```python
from build123d import *

# Parameters (mm, degrees)
BOSS_EXTRUDE2_DEPTH  = 18.5
M3_CLEARANCE_HOLE1_D = 3.2
BOSS_EXTRUDE3_REACH  = 43.692
CUT_EXTRUDE1_REACH   = 43.692
FILLET1_R            = 2
FILLET2_R            = 1


# Some blends are built 0.0001 mm under size
with BuildPart() as part:
    # Sketch2 → Boss-Extrude2 (new, symmetric)
    with BuildSketch(Plane.XY):
        with BuildLine():
            Line((-8, 0), (-8, -9))
            Line((-8, -9), (-16, -9))
            Line((-16, -9), (-16, -7))
            Line((-16, -7), (-10, -7))
            Line((-10, -7), (-10, 0))
            ThreePointArc((-10, 0), (0, 10), (10, 0))
            Line((10, 0), (10, -7))
            Line((10, -7), (16, -7))
            Line((16, -7), (16, -9))
            Line((16, -9), (8, -9))
            Line((8, -9), (8, 0))
            ThreePointArc((8, 0), (0, 8), (-8, 0))
        make_face()
    extrude(amount=BOSS_EXTRUDE2_DEPTH, both=True)

    # M3 Clearance Hole1 (through all)
    with Locations(Plane(origin=(0, -7, 0), x_dir=(1, 0, 0), z_dir=(0, 1, 0))):
        with Locations((-13, 14.25), (13, 14.25), (13, -14.25), (-13, -14.25)):
            Hole(M3_CLEARANCE_HOLE1_D / 2)

    # Sketch6 → Boss-Extrude3 (add, up to next)
    with BuildSketch(Plane(origin=(20, 0, 0), x_dir=(0, 0, -1), z_dir=(1, 0, 0)), mode=Mode.PRIVATE) as boss_extrude3_sk1:
        with BuildLine():
            Line((-8, 0), (-8, -9))
            Line((-8, -9), (-10, -9))
            Line((-10, -9), (-10, 0))
            ThreePointArc((-10, 0), (0, 10), (10, 0))
            Line((10, 0), (10, -9))
            Line((10, -9), (8, -9))
            Line((8, -9), (8, 0))
            ThreePointArc((8, 0), (0, 8), (-8, 0))
        make_face()
    boss_extrude3_tool1 = extrude(boss_extrude3_sk1.sketch, amount=-BOSS_EXTRUDE3_REACH, mode=Mode.PRIVATE) - part.part
    add(boss_extrude3_tool1.solids().sort_by_distance((20, -4.5, -9.724138))[0])

    # Sketch7 → Cut-Extrude1 (cut, up to next)
    with BuildSketch(Plane(origin=(20, 0, 0), x_dir=(0, 0, -1), z_dir=(1, 0, 0)), mode=Mode.PRIVATE) as cut_extrude1_sk1:
        with BuildLine():
            Line((8, 0), (8, -7))
            Line((8, -7), (8, -9))
            Line((8, -9), (-8, -9))
            Line((-8, -9), (-8, -7))
            Line((-8, -7), (-8, 0))
            ThreePointArc((-8, 0), (0, 8), (8, 0))
        make_face()
    cut_extrude1_tool1 = extrude(cut_extrude1_sk1.sketch, amount=-CUT_EXTRUDE1_REACH, mode=Mode.PRIVATE) & part.part
    add(cut_extrude1_tool1.solids().sort_by_distance((20, -1.254102, 0))[0], mode=Mode.SUBTRACT)

    # Fillet1
    fillet1_edges = [part.edges().sort_by_distance(p)[0] for p in [
        (16, -8, -10),
        (16, -8, 10),
        (16, -8, 18.5),
        (16, -8, -18.5),
        (-16, -8, 18.5),
        (-16, -8, -18.5),
        (20, -4.5, 10),
        (20, 10, 0),
        (20, -4.5, -10),
        (10, -3.5, -18.5),
        (-10, -3.5, -18.5),
        (10, -3.5, 18.5),
        (-10, -3.5, 18.5),
        (0, 10, -18.5),
        (0, 10, 18.5),
    ]]
    fillet(fillet1_edges, radius=FILLET1_R - 0.0001)  # a hair under: the kernel refuses the full size

    # Fillet2
    # the kernel refuses this fillet: 1 mm, written as the material it adds along each edge
    with BuildSketch(Plane(origin=(-10, -7, 16.5001), x_dir=(0, 1, 0), z_dir=(0, 0, -1))) as fillet2_piece_1:
        with BuildLine():
            CenterArc((FILLET2_R, -FILLET2_R), FILLET2_R, 90, 90)
            Line((0, -FILLET2_R), (0, 0))
            Line((0, 0), (FILLET2_R, 0))
        make_face()
    extrude(amount=33.0002)
    with BuildSketch(Plane(origin=(10, -7, 16.5001), x_dir=(0, 1, 0), z_dir=(0, 0, -1)), Plane(origin=(10, -7, -10), x_dir=(0, 1, 0), z_dir=(0, 0, -1))) as fillet2_piece_2:
        with BuildLine():
            CenterArc((FILLET2_R, FILLET2_R), FILLET2_R, 180, 90)
            Line((0, FILLET2_R), (0, 0))
            Line((0, 0), (FILLET2_R, 0))
        make_face()
    extrude(amount=6.5001)
    with BuildSketch(Plane(origin=(8.0001, -7, -16.5001), x_dir=(1, 0, 0), z_dir=(0, 0, 1))) as fillet2_piece_3_section:
        with BuildLine():
            CenterArc((1.9999 + FILLET2_R, FILLET2_R), FILLET2_R, 180, 90)
            Line((1.9999, FILLET2_R), (1.9999, 0))
            Line((1.9999, 0), (1.9999 + FILLET2_R, 0))
        make_face()
    fillet2_piece_3 = revolve(axis=Axis((8.0001, -7, -16.5001), (0, 1, 0)), revolution_arc=161.652077223, mode=Mode.PRIVATE)
    fillet2_piece_3 = split(fillet2_piece_3, bisect_by=Plane(origin=(10.2121031, -6.837361474, -18.5), z_dir=(0, 0, 1)), keep=Keep.TOP, mode=Mode.PRIVATE)
    fillet2_piece_3 = split(fillet2_piece_3, bisect_by=Plane(origin=(8, -6.837361474, -17.073760291), z_dir=(1, 0, 0)), keep=Keep.TOP, mode=Mode.PRIVATE)
    add(fillet2_piece_3)
    with BuildSketch(Plane(origin=(-8.0001, -7, -16.5001), x_dir=(-1, 0, 0), z_dir=(0, 0, 1))) as fillet2_piece_4_section:
        with BuildLine():
            CenterArc((1.9999 + FILLET2_R, -FILLET2_R), FILLET2_R, 90, 90)
            Line((1.9999 + FILLET2_R, 0), (1.9999, 0))
            Line((1.9999, 0), (1.9999, -FILLET2_R))
        make_face()
    fillet2_piece_4 = revolve(axis=Axis((-8.0001, -7, -16.5001), (0, -1, 0)), revolution_arc=161.652077223, mode=Mode.PRIVATE)
    fillet2_piece_4 = split(fillet2_piece_4, bisect_by=Plane(origin=(-8, -6.727847021, -17.962226861), z_dir=(-1, 0, 0)), keep=Keep.TOP, mode=Mode.PRIVATE)
    fillet2_piece_4 = split(fillet2_piece_4, bisect_by=Plane(origin=(-9.462226887, -6.727847021, -18.5), z_dir=(0, 0, 1)), keep=Keep.TOP, mode=Mode.PRIVATE)
    add(fillet2_piece_4)
    with BuildSketch(Plane(origin=(8.0001, -7, 16.5001), x_dir=(-0.949162519062451, 0, 0.3147864552470806), z_dir=(-0.3147864552470806, 0, -0.949162519062451))) as fillet2_piece_5_section:
        with BuildLine():
            CenterArc((1.9999 + FILLET2_R, FILLET2_R), FILLET2_R, 180, 90)
            Line((1.9999, FILLET2_R), (1.9999, 0))
            Line((1.9999, 0), (1.9999 + FILLET2_R, 0))
        make_face()
    fillet2_piece_5 = revolve(axis=Axis((8.0001, -7, 16.5001), (0, 1, 0)), revolution_arc=161.652077223, mode=Mode.PRIVATE)
    fillet2_piece_5 = split(fillet2_piece_5, bisect_by=Plane(origin=(9.462226477, -6.727846247, 18.5), z_dir=(0, 0, -1)), keep=Keep.TOP, mode=Mode.PRIVATE)
    fillet2_piece_5 = split(fillet2_piece_5, bisect_by=Plane(origin=(8, -6.727846247, 17.962227025), z_dir=(1, 0, 0)), keep=Keep.TOP, mode=Mode.PRIVATE)
    add(fillet2_piece_5)
    with BuildSketch(Plane(origin=(-8.0001, -7, 16.5001), x_dir=(0.949162519062451, 0, 0.3147864552470806), z_dir=(0.3147864552470806, 0, -0.949162519062451))) as fillet2_piece_6_section:
        with BuildLine():
            CenterArc((1.9999 + FILLET2_R, -FILLET2_R), FILLET2_R, 90, 90)
            Line((1.9999 + FILLET2_R, 0), (1.9999, 0))
            Line((1.9999, 0), (1.9999, -FILLET2_R))
        make_face()
    fillet2_piece_6 = revolve(axis=Axis((-8.0001, -7, 16.5001), (0, -1, 0)), revolution_arc=161.652077223, mode=Mode.PRIVATE)
    fillet2_piece_6 = split(fillet2_piece_6, bisect_by=Plane(origin=(-9.462226765, -6.727846718, 18.5), z_dir=(0, 0, -1)), keep=Keep.TOP, mode=Mode.PRIVATE)
    fillet2_piece_6 = split(fillet2_piece_6, bisect_by=Plane(origin=(-8, -6.727846718, 17.962226739), z_dir=(-1, 0, 0)), keep=Keep.TOP, mode=Mode.PRIVATE)
    add(fillet2_piece_6)


solid = part.part
```
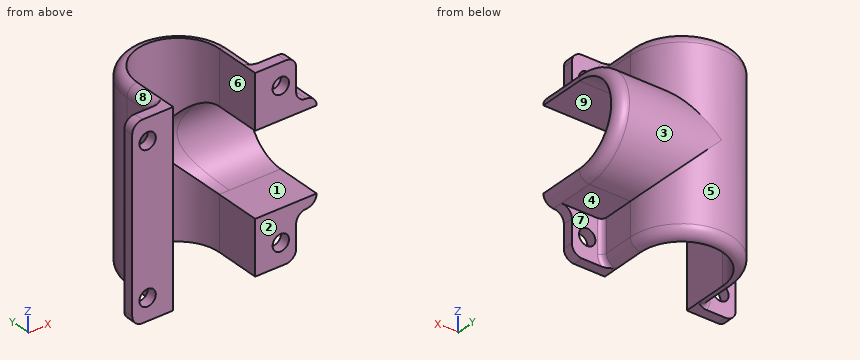
Input: part model. Units: mm. Frame: model coordinates. Face numbers are marked on the shaded views. A direction names the side the tool comes from. Coordinates: 2 decimals unless noted, no trailing zeros. Write each loop counter-clockwise with the first axis right and the second up, starting at its lowest first coordinate (ties: lowest second). Pieces come first, ordered by that corner, then holes.
1) Section D-D on x = 15.5. Output: boundary loops of the cut face in (y, z), and give its area (3 significant figures).
2) Section B-B on y = -2.5. State how many separate pieces and enclosed holes the cut face has, and give its area (3 significant figures).
3) Pin query (flat end, axial travel): pin 1 Ø2.5 at (y, z) = (-5, -2.5) entering from +X; pin 2 Ø4 at (x, z) = (13, 13) entering from +Y; pin 3 Ø3 at (x, z) = (13, -14.25) entering from +Y; pin 4 Ø1 at (y, z) = (-4.5, 3) entering from -X. Return the tip coordinate at first contact, or that it passes through.
4) Set-up query: the marked faces 5, 6, 7, 8 and 9. Return all of +Z, -Z, +X, -X, +Y, -Y with unobstructed straight access to the full face (end or side cutting, diameter ignored); none if empty.
5) Material intervals for line 1 along X through (y, z) = (-8.3, 14.25); line 2 along Z through (x, y) = (-13, -7.65); line 3 along Z through (x, y) = (13, -8.1), sorted ascending.
6) Mould query, pull axis Z, two halves, no side actions, for the marked faces 1, 2, 3 and 4. Classes: pulls with the +Z half, pulls with the -Z half, needs draft (parallel to the pull), parting line crosses it, or undercut.
7) Section C-C on z = -14.25. Output: boundary loops of the cut face in (x, y), and give its area (3 significant figures).
8) Section A-A on x = -13. Output: boundary loops of the cut face in (y, z).
Check result:
1. outline: (-9, -17.82) - (-7, -17.82) - (-7, -10) - (0, -10) arc R10 ccw to (0, 10) - (-7, 10) - (-7, 17.82) - (-9, 17.82) - (-9, 8) - (0, 8) arc R8 cw to (0, -8) - (-9, -8) - close
1. area: 124 mm2
2. separate pieces: 3
2. enclosed holes: 0
2. area: 151 mm2
3. pin 1: stops at x = -8
3. pin 2: stops at y = -7
3. pin 3: passes through
3. pin 4: stops at x = -10
4. face 5: +Y
4. face 6: +Z, -Z, -Y
4. face 7: -Z, +X, +Y
4. face 8: +Z, -X, +Y
4. face 9: +X, -Y
5. line 1: x = -16 to -14.6, -11.4 to -8, 8 to 11.4, 14.6 to 16
5. line 2: z = -18.5 to -15.85, -12.65 to 12.65, 15.85 to 18.5
5. line 3: z = -18.5 to -15.85, -12.65 to -8, 8 to 12.65, 15.85 to 18.5
6. face 1: undercut
6. face 2: needs draft
6. face 3: parting line crosses it
6. face 4: pulls with the -Z half
7. outline: (-16, -9) - (-14.6, -9) - (-14.6, -7) - (-16, -7) - close; (-11.4, -9) - (-8, -9) - (-8, 0) arc R8 cw to (8, 0) - (8, -9) - (11.4, -9) - (11.4, -7) - (11, -7) arc R1 cw to (10, -6) - (10, 0) arc R10 ccw to (-10, 0) - (-10, -6) arc R1 cw to (-11, -7) - (-11.4, -7) - close; (14.6, -9) - (16, -9) - (16, -7) - (14.6, -7) - close
7. area: 104 mm2
8. outline: (-9, -18.5) - (-7, -18.5) - (-7, -15.85) - (-9, -15.85) - close; (-9, -12.65) - (-7, -12.65) - (-7, 12.65) - (-9, 12.65) - close; (-9, 15.85) - (-7, 15.85) - (-7, 18.5) - (-9, 18.5) - close
